```python
from build123d import *

# Parameters (mm, degrees)
SKETCH_1_W          = 120
SKETCH_1_H          = 60
EXTRUDE_1_DEPTH     = 5
CUT_EXTRUDE_1_REACH = 115.997
SKETCH_2_R          = 1.65
CUT_EXTRUDE_2_REACH = 115.997
SKETCH_4_R          = 1.6
FILLET_1_R          = 1


with BuildPart() as part:
    # 草图1 → 凸台-拉伸1 (new body)
    with BuildSketch(Plane.XY):
        with Locations((-40, -24.5)):
            Rectangle(SKETCH_1_W, SKETCH_1_H)
    extrude(amount=EXTRUDE_1_DEPTH)

    # 草图2 → 切除-拉伸1 (cut, up to next)
    with BuildSketch(Plane.XY.offset(5), mode=Mode.PRIVATE) as cut_extrude_1_sk1:
        with Locations((-25, -13)):
            Circle(SKETCH_2_R)
    cut_extrude_1_tool1 = extrude(cut_extrude_1_sk1.sketch, amount=-CUT_EXTRUDE_1_REACH, mode=Mode.PRIVATE) & part.part
    # 草图2 → 切除-拉伸1 (cut, up to next)
    with BuildSketch(Plane.XY.offset(5), mode=Mode.PRIVATE) as cut_extrude_1_sk2:
        with Locations((-50, -24.5)):
            Circle(SKETCH_2_R)
    cut_extrude_1_tool2 = extrude(cut_extrude_1_sk2.sketch, amount=-CUT_EXTRUDE_1_REACH, mode=Mode.PRIVATE) & part.part
    # 草图2 → 切除-拉伸1 (cut, up to next)
    with BuildSketch(Plane.XY.offset(5), mode=Mode.PRIVATE) as cut_extrude_1_sk3:
        with Locations((-25, -36)):
            Circle(SKETCH_2_R)
    cut_extrude_1_tool3 = extrude(cut_extrude_1_sk3.sketch, amount=-CUT_EXTRUDE_1_REACH, mode=Mode.PRIVATE) & part.part
    add(cut_extrude_1_tool1.solids().sort_by_distance((-25, -13, 5))[0], mode=Mode.SUBTRACT)
    add(cut_extrude_1_tool2.solids().sort_by_distance((-50, -24.5, 5))[0], mode=Mode.SUBTRACT)
    add(cut_extrude_1_tool3.solids().sort_by_distance((-25, -36, 5))[0], mode=Mode.SUBTRACT)

    # 草图4 → 切除-拉伸2 (cut, up to next)
    with BuildSketch(Plane(origin=(0, 0, 0), x_dir=(-1, 0, 0), z_dir=(0, 0, -1)), mode=Mode.PRIVATE) as cut_extrude_2_sk1:
        with Locations((90, 0)):
            Circle(SKETCH_4_R)
    cut_extrude_2_tool1 = extrude(cut_extrude_2_sk1.sketch, amount=-CUT_EXTRUDE_2_REACH, mode=Mode.PRIVATE) & part.part
    # 草图4 → 切除-拉伸2 (cut, up to next)
    with BuildSketch(Plane(origin=(0, 0, 0), x_dir=(-1, 0, 0), z_dir=(0, 0, -1)), mode=Mode.PRIVATE) as cut_extrude_2_sk2:
        with Locations((70, 0)):
            Circle(SKETCH_4_R)
    cut_extrude_2_tool2 = extrude(cut_extrude_2_sk2.sketch, amount=-CUT_EXTRUDE_2_REACH, mode=Mode.PRIVATE) & part.part
    # 草图4 → 切除-拉伸2 (cut, up to next)
    with BuildSketch(Plane(origin=(0, 0, 0), x_dir=(-1, 0, 0), z_dir=(0, 0, -1)), mode=Mode.PRIVATE) as cut_extrude_2_sk3:
        with Locations((70, -50)):
            Circle(SKETCH_4_R)
    cut_extrude_2_tool3 = extrude(cut_extrude_2_sk3.sketch, amount=-CUT_EXTRUDE_2_REACH, mode=Mode.PRIVATE) & part.part
    # 草图4 → 切除-拉伸2 (cut, up to next)
    with BuildSketch(Plane(origin=(0, 0, 0), x_dir=(-1, 0, 0), z_dir=(0, 0, -1)), mode=Mode.PRIVATE) as cut_extrude_2_sk4:
        with Locations((90, -50)):
            Circle(SKETCH_4_R)
    cut_extrude_2_tool4 = extrude(cut_extrude_2_sk4.sketch, amount=-CUT_EXTRUDE_2_REACH, mode=Mode.PRIVATE) & part.part
    # 草图4 → 切除-拉伸2 (cut, up to next)
    with BuildSketch(Plane(origin=(0, 0, 0), x_dir=(-1, 0, 0), z_dir=(0, 0, -1)), mode=Mode.PRIVATE) as cut_extrude_2_sk5:
        with Locations((10, -50)):
            Circle(SKETCH_4_R)
    cut_extrude_2_tool5 = extrude(cut_extrude_2_sk5.sketch, amount=-CUT_EXTRUDE_2_REACH, mode=Mode.PRIVATE) & part.part
    # 草图4 → 切除-拉伸2 (cut, up to next)
    with BuildSketch(Plane(origin=(0, 0, 0), x_dir=(-1, 0, 0), z_dir=(0, 0, -1)), mode=Mode.PRIVATE) as cut_extrude_2_sk6:
        with Locations((-10, -50)):
            Circle(SKETCH_4_R)
    cut_extrude_2_tool6 = extrude(cut_extrude_2_sk6.sketch, amount=-CUT_EXTRUDE_2_REACH, mode=Mode.PRIVATE) & part.part
    # 草图4 → 切除-拉伸2 (cut, up to next)
    with BuildSketch(Plane(origin=(0, 0, 0), x_dir=(-1, 0, 0), z_dir=(0, 0, -1)), mode=Mode.PRIVATE) as cut_extrude_2_sk7:
        with Locations((-10, 0)):
            Circle(SKETCH_4_R)
    cut_extrude_2_tool7 = extrude(cut_extrude_2_sk7.sketch, amount=-CUT_EXTRUDE_2_REACH, mode=Mode.PRIVATE) & part.part
    # 草图4 → 切除-拉伸2 (cut, up to next)
    with BuildSketch(Plane(origin=(0, 0, 0), x_dir=(-1, 0, 0), z_dir=(0, 0, -1)), mode=Mode.PRIVATE) as cut_extrude_2_sk8:
        with Locations((10, 0)):
            Circle(SKETCH_4_R)
    cut_extrude_2_tool8 = extrude(cut_extrude_2_sk8.sketch, amount=-CUT_EXTRUDE_2_REACH, mode=Mode.PRIVATE) & part.part
    add(cut_extrude_2_tool1.solids().sort_by_distance((-90, 0, 0))[0], mode=Mode.SUBTRACT)
    add(cut_extrude_2_tool2.solids().sort_by_distance((-70, 0, 0))[0], mode=Mode.SUBTRACT)
    add(cut_extrude_2_tool3.solids().sort_by_distance((-70, -50, 0))[0], mode=Mode.SUBTRACT)
    add(cut_extrude_2_tool4.solids().sort_by_distance((-90, -50, 0))[0], mode=Mode.SUBTRACT)
    add(cut_extrude_2_tool5.solids().sort_by_distance((-10, -50, 0))[0], mode=Mode.SUBTRACT)
    add(cut_extrude_2_tool6.solids().sort_by_distance((10, -50, 0))[0], mode=Mode.SUBTRACT)
    add(cut_extrude_2_tool7.solids().sort_by_distance((10, 0, 0))[0], mode=Mode.SUBTRACT)
    add(cut_extrude_2_tool8.solids().sort_by_distance((-10, 0, 0))[0], mode=Mode.SUBTRACT)

    # 圆角1
    fillet_1_edges = [part.edges().sort_by_distance(p)[0] for p in [
        (20, -54.5, 2.5),
        (-100, -54.5, 2.5),
        (-100, 5.5, 2.5),
        (20, 5.5, 2.5),
    ]]
    fillet(fillet_1_edges, radius=FILLET_1_R)


solid = part.part
```
CAD build for the part. Positions are in the model's coordinates, mm. Coordinates: 2 decimals unless noted, no trailing zeros. Order: outer loops, then holes, each group sorted by start corner. A loop starts at its lowest first (then second) coordinate and runs counter-clockwise, first axis right, second up. Notation, with made-up numbers: (46, -15) - (75, -15) arc R35 ccw to (75, 24) - close; hole circle Ø2 at (24, 77). An arc over 180 degrees is marked (long way). Use a Markdown table: item, result. Add a question column.
(1) Saw through at B-B (y = 0). Give the cut face in (x, z).
(2) Saw through at C-C (y = -36). Give the cut face in (x, z), then the cut area to 4 significant figures.
(3) Flat gauge pin, fed straight in: pin 1 (4 mm diameter, centred on x = -10, y = 0, fed in from +Z). Where does the tip first touch, or does it go through?
(4) Saw through at D-D (x = -25). Give the cut face in (y, z), then the cut area to 3 significant figures.
(5) Saw through at A-A (x = 10). Give the cut face in (y, z).
(6) Pull direction Y, two halves, no side cores. Call faces 1 (the face through (-41, 5.5, 2)), 2 (the face through (-41, -24, 5)), 3 (the face through (-26.65, -12.93, 2.54)): +Y half, -Y half, draft (parallel to the pull), parting line (faces both ways), or undercut.
(7) Drill centre lines: line 1 along Y through (x, z) = (-70, 2.9); line 2 along X through (y, z) = (-24, 1.05); line 3 along Y through (x, z) = (-50, 3.6). Where is each one in solid material? Low to high. Write a range as [from, to].
Solved:
| question | item | result |
|---|---|---|
| 1 | outline | (-100, 0) - (-91.6, 0) - (-91.6, 5) - (-100, 5) - close; (-88.4, 0) - (-71.6, 0) - (-71.6, 5) - (-88.4, 5) - close; (-68.4, 0) - (-11.6, 0) - (-11.6, 5) - (-68.4, 5) - close; (-8.4, 0) - (8.4, 0) - (8.4, 5) - (-8.4, 5) - close; (11.6, 0) - (20, 0) - (20, 5) - (11.6, 5) - close |
| 2 | outline | (-100, 0) - (-26.65, 0) - (-26.65, 5) - (-100, 5) - close; (-23.35, 0) - (20, 0) - (20, 5) - (-23.35, 5) - close |
| 2 | area | 583.5 mm² |
| 3 | pin 1 | stops at z = 5 |
| 4 | outline | (-54.5, 0) - (-37.65, 0) - (-37.65, 5) - (-54.5, 5) - close; (-34.35, 0) - (-14.65, 0) - (-14.65, 5) - (-34.35, 5) - close; (-11.35, 0) - (5.5, 0) - (5.5, 5) - (-11.35, 5) - close |
| 4 | area | 267 mm² |
| 5 | outline | (-54.5, 0) - (-51.6, 0) - (-51.6, 5) - (-54.5, 5) - close; (-48.4, 0) - (-1.6, 0) - (-1.6, 5) - (-48.4, 5) - close; (1.6, 0) - (5.5, 0) - (5.5, 5) - (1.6, 5) - close |
| 6 | face 1 | +Y half |
| 6 | face 2 | draft |
| 6 | face 3 | undercut |
| 7 | line 1 | y = [-54.5, -51.6], [-48.4, -1.6], [1.6, 5.5] |
| 7 | line 2 | x = [-100, -51.57], [-48.43, 20] |
| 7 | line 3 | y = [-54.5, -26.15], [-22.85, 5.5] |
